Part print with two shaded views. Sizes in mm from the minimum x, y, z corner. A direction names the side the tool comes from. Round coordinates to 2 decimals unless told otherwise and drop trailing zeros. Loops run counter-clockwise (first coordinate to the right, second up) from the corner with the lowest first, then second, coordinate; pieces in that order, holes last.
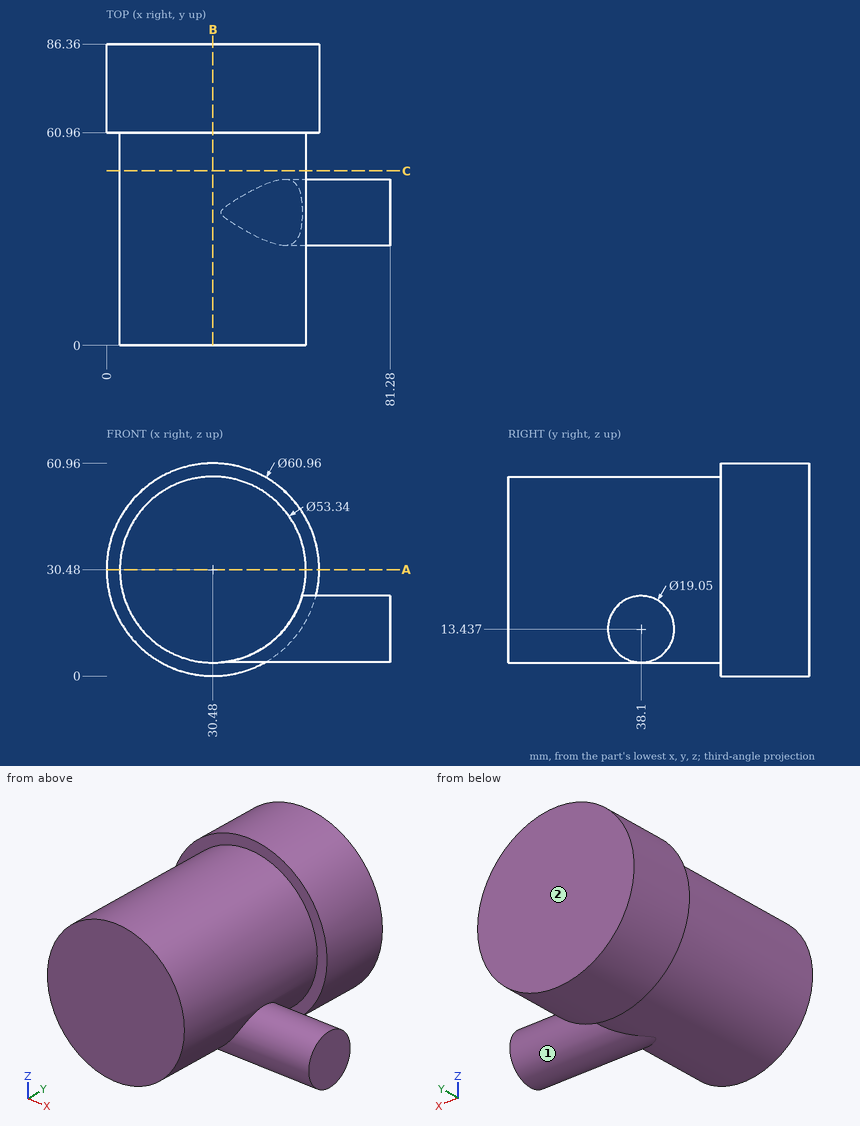
Item 1: Cut at B-B (x = 30.48). List the corners of the cut face in (y, z).
Verdict:
outline: (0, 3.81) - (60.96, 3.81) - (60.96, 0) - (86.36, 0) - (86.36, 60.96) - (60.96, 60.96) - (60.96, 57.15) - (0, 57.15) - close
Item 2: Cut at A-A (z = 30.48). List the corners of the cut face in (x, y).
Verdict:
outline: (0, 60.96) - (3.81, 60.96) - (3.81, 0) - (57.15, 0) - (57.15, 60.96) - (60.96, 60.96) - (60.96, 86.36) - (0, 86.36) - close
Item 3: Cut at C-C (y = 50). List the corners of the cut face in (x, z).
Verdict:
outline: circle Ø53.34 at (30.48, 30.48)
Item 4: 3-axis set-ups, long thin cutter, end or side, ignore diameter. For the marked faces 1 and 2: which of +Z, -Z, +X, -X, +Y, -Y reach the whole face in a straight line?
Verdict:
face 1: +X
face 2: +Z, -Z, +X, -X, +Y
Item 5: Flat gauge pins, fed straight in: P1, Ø4, axis at x = 55, z = 49, coming from the -Y side; P2, Ø8, axis at y = 19, z = 37, coming from the +X side; P3, Ø3, axis at x = 36.5, y = 58.5, coming from the +Z side. Where does each tip first touch, or does it go through?
Verdict:
P1: stops at y = 60.96
P2: stops at x = 57.03
P3: stops at z = 56.76
Item 6: Wall check: L1, parallel to Y at x = 51.5, z = 14; L2, parallel to Y at x = 19, z = 4; L3, parallel to X at y = 54, z = 30 (1 decimal). Give the ranges that are in metal, low to high.
Verdict:
L1: y = 28.59 to 47.61, 60.96 to 86.36
L2: y = 60.96 to 86.36
L3: x = 3.8 to 57.1
